CAD build for the part. Positions are in the model's coordinates, mm. Face numbers are marked on the shaded views. A direction names the side the tool comes from. Give positions to 0.01 mm unless a question says otherwise; leave off trailing zeros. Order: outer loops, then holes, each group sorted by start corner. A loop starts at its lowest first (then second) coordinate and runs counter-clockwise, first axis right, second up. Notation, with made-up numbers: (8.25, 41) -> (39.25, 41) arc R37 cw to (39.25, 79) -> close; hole circle Ø9 at (85, 21). An arc over 180 degrees is marked (long way). Answer as CSV lines item,"result".
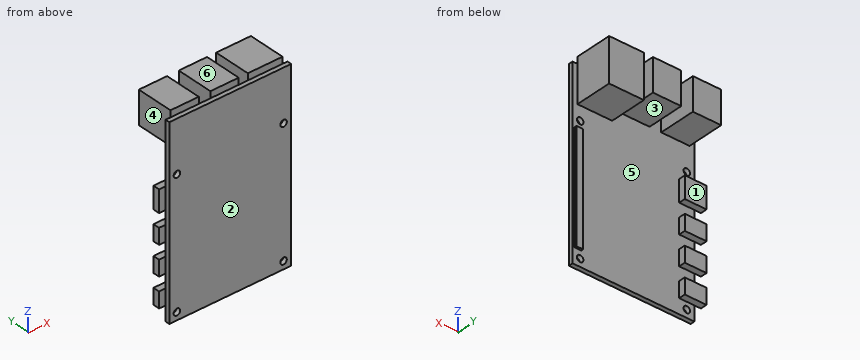
```python
from build123d import *

# Parameters (mm, degrees)
SKETCH1_W           = 56
SKETCH1_H           = 85
SKETCH1_R           = 1.5
BOSS_EXTRUDE1_DEPTH = 2
SKETCH2_W           = 3
SKETCH2_H           = 50.7
BOSS_EXTRUDE2_DEPTH = 1
SKETCH3_W           = 13
SKETCH3_H           = 15
SKETCH3_W_2         = 15.95
SKETCH3_H_2         = 20
BOSS_EXTRUDE3_DEPTH = 17
SKETCH4_W           = 10
SKETCH4_H           = 7.2
SKETCH4_H_2         = 10
BOSS_EXTRUDE4_DEPTH = 3


with BuildPart() as part:
    # Sketch1 → Boss-Extrude1 (new body)
    with BuildSketch(Plane(origin=(0, 0, 0), x_dir=(1, 0, 0), z_dir=(0, 1, 0))):
        Rectangle(SKETCH1_W, SKETCH1_H)
        with Locations(Location((-24.5, 39, 0), (0, 0, 270))):
            Circle(SKETCH1_R, mode=Mode.SUBTRACT)
        with Locations(Location((24.5, 39, 0), (0, 0, 270))):
            Circle(SKETCH1_R, mode=Mode.SUBTRACT)
        with Locations(Location((-24.5, -19, 0), (0, 0, 270))):
            Circle(SKETCH1_R, mode=Mode.SUBTRACT)
        with Locations(Location((24.5, -19, 0), (0, 0, 270))):
            Circle(SKETCH1_R, mode=Mode.SUBTRACT)
    extrude(amount=BOSS_EXTRUDE1_DEPTH)

    # Sketch2 → Boss-Extrude2 (add)
    with BuildSketch(Plane(origin=(0, 2, 0), x_dir=(1, 0, 0), z_dir=(0, 1, 0))):
        with Locations((25.5, 10.05)):
            Rectangle(SKETCH2_W, SKETCH2_H)
    extrude(amount=BOSS_EXTRUDE2_DEPTH)

    # Sketch3 → Boss-Extrude3 (add)
    with BuildSketch(Plane(origin=(0, 2, 0), x_dir=(1, 0, 0), z_dir=(0, 1, 0))):
        with Locations((-19.25, -38)):
            Rectangle(SKETCH3_W, SKETCH3_H)
        with Locations((-0.9, -38)):
            Rectangle(SKETCH3_W, SKETCH3_H)
        with Locations((17.775, -35.5)):
            Rectangle(SKETCH3_W_2, SKETCH3_H_2)
    extrude(amount=BOSS_EXTRUDE3_DEPTH)

    # Sketch4 → Boss-Extrude4 (add)
    with BuildSketch(Plane(origin=(0, 2, 0), x_dir=(1, 0, 0), z_dir=(0, 1, 0))):
        with Locations((-26, 32.1)):
            Rectangle(SKETCH4_W, SKETCH4_H)
        with Locations((-26, 5.3)):
            Rectangle(SKETCH4_W, SKETCH4_H)
        with Locations((-26, -9.5)):
            Rectangle(SKETCH4_W, SKETCH4_H_2)
        with Locations((-26, 18.7)):
            Rectangle(SKETCH4_W, SKETCH4_H)
    extrude(amount=BOSS_EXTRUDE4_DEPTH)


solid = part.part
```
1) Band-saw the part on B-B, the plane x = -24.5. Give the number of separate pieces and of enclosed holes in the cut face, then the cut area to 3 significant figures.
Data:
separate pieces,"3"
enclosed holes,"0"
area,"508 mm2"
2) Band-saw the part on C-C, the plane z = -39. Write the cut outline in (x, y).
Data:
outline,"(-28, 0) -> (-26, 0) -> (-26, 2) -> (-28, 2) -> close; (-23, 0) -> (23, 0) -> (23, 2) -> (-23, 2) -> close; (26, 0) -> (28, 0) -> (28, 2) -> (26, 2) -> close"
3) Band-saw the part on A-A, the plane y = 12. Write the cut outline in (x, z).
Data:
outline,"(-25.75, 30.5) -> (-12.75, 30.5) -> (-12.75, 45.5) -> (-25.75, 45.5) -> close; (-7.4, 30.5) -> (5.6, 30.5) -> (5.6, 45.5) -> (-7.4, 45.5) -> close; (9.8, 25.5) -> (25.75, 25.5) -> (25.75, 45.5) -> (9.8, 45.5) -> close"
4) Wall check: line 1 along X through (y, z) = (0.4, -39); line 2 along Z through (x, y) = (-3, 10); line 3 along Y through (x, z) = (-19, -10.5). Give the ranges that are in metal, low to high. Write a range as [from, to].
Data:
line 1,"x = [-28, -26], [-23, 23], [26, 28]"
line 2,"z = [30.5, 45.5]"
line 3,"y = [0, 2]"
5) Pull direction X, two halves, no side cores. Call the marked faces 4, 5 and 6: pulls with the +X half, pulls with the -X half, needs draft (parallel to the pull), parting line crosses it, or undercut.
Data:
face 4,"pulls with the -X half"
face 5,"undercut"
face 6,"needs draft"
6) Band-saw the part on D-D, the plane x = 14.5. Write the cut outline in (y, z).
Data:
outline,"(0, -42.5) -> (2, -42.5) -> (2, 25.5) -> (19, 25.5) -> (19, 45.5) -> (2, 45.5) -> (2, 42.5) -> (0, 42.5) -> close"
7) Pin check, flat tips, straight feed: P1, Ø1.5, axis at x = 0.5, z = 44, coming from the -Y side; P2, Ø1.8, axis at x = 24.5, z = -39, coming from the -Y side; P3, Ø1.5, axis at x = -24.5, z = -4.5, coming from the +Y side; P4, Ø10.5, axis at x = -16, y = 12.5, coming from the -Z side. Stop position of each tip, or through.
Data:
P1,"stops at y = 2"
P2,"passes through"
P3,"stops at y = 5"
P4,"stops at z = 30.5"
8) Which spindle directions (+Z, -Z, +X, -X, +Y, -Y) get a long thin tool onto all of the face, cutting with end or side? Do the marked faces 1, 2 and 3. Say none if no direction does.
Data:
face 1,"-Z, +X, -X, +Y"
face 2,"+Z, -Z, +X, -X, -Y"
face 3,"-Z, -X, +Y"
